Here's how the part is built. I have some questions about the finished solid (model axes, mm). Face numbers are marked on the shaded views. A direction names the side the tool comes from. Coordinates: 2 decimals unless noted, no trailing zeros. Write each loop counter-clockwise with the first axis right and the second up, starting at its lowest first coordinate (ties: lowest second). Pieces come first, ordered by that corner, then holes.
Item 1: I want a section at C-C (y = -480.5). Please give me the cut outline in (x, z), and give its area (3 significant figures).
Item 2: For the marked faces 1 and 2, which set-ups out of +Z, -Z, +X, -X, +Y, -Y let a thin tool reach every point of the face, with its end or its side?
Item 3: I want a section at D-D (z = 128.5). Please give me the cut outline in (x, y).
Item 4: Please list where these lines run through material, in increasing order: line 1 (Z direction, x = 0, y = -758); line 2 (Y direction, x = 2, z = -102.5); line 3 (Z direction, x = 10.5, y = -552).
Item 5: I'm going to push flat-ended pins straight in: P1, Ø10, axis at x = -19.5, z = -113, coming from the +Y side; P2, Ø8, axis at x = -14, y = -556.5, coming from the +Z side; P3, Ø6, axis at y = -424, z = -17.5, coming from the -X side. Where does each tip first touch, or does it pass through?
Item 6: I want a section at A-A (x = 0). Please give me the cut outline in (y, z), and give its area (3 significant figures).
Item 7: I want a section at B-B (z = 0). Please give me the cut outline in (x, y), and give its area (3 significant figures).
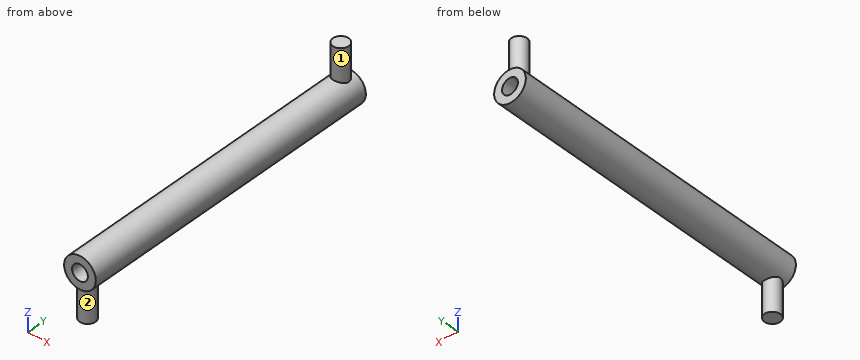
from build123d import *

# Parameters (mm, degrees)
F0_R     = 50
F0_R_2   = 25
F3_DEPTH = 1000
F4_R     = 25
F5_DEPTH = 125
F6_R     = 25
F7_DEPTH = 125


with BuildPart() as f3:
    # F0 (on Front) → F3 (new body)
    with BuildSketch(Plane.XZ):
        Circle(F0_R)
        Circle(F0_R_2, mode=Mode.SUBTRACT)
    extrude(amount=F3_DEPTH)

    # F4 (on offset) → F5 (join)
    with BuildSketch(Plane.XY.offset(-25)):
        with Locations((0, -971.540222)):
            Circle(F4_R)
    extrude(amount=-F5_DEPTH)

    # F6 (on offset) → F7 (join)
    with BuildSketch(Plane.XY.offset(25)):
        with Locations((0, -34.047124)):
            Circle(F6_R)
    extrude(amount=F7_DEPTH)


solid = f3.part
Answer:
1. outline: circle Ø100 at (0, 0); hole circle Ø50 at (0, 0)
1. area: 5,890 mm2
2. face 1: +Z
2. face 2: -Z
3. outline: circle Ø50 at (0, -34.05)
4. line 1: z = -50 to -25, 25 to 50
4. line 2: y = -996.46 to -946.62
4. line 3: z = -48.89 to -22.69, 22.69 to 48.89
5. P1: stops at y = -951.17
5. P2: stops at z = 48.99
5. P3: stops at x = -47.85
6. outline: (-1000, -50) - (-996.54, -50) - (-996.54, -150) - (-946.54, -150) - (-946.54, -50) - (0, -50) - (0, -25) - (-1000, -25) - close; (-1000, 25) - (0, 25) - (0, 50) - (-9.05, 50) - (-9.05, 150) - (-59.05, 150) - (-59.05, 50) - (-1000, 50) - close
6. area: 60,000 mm2
7. outline: (-50, -1000) - (-25, -1000) - (-25, 0) - (-50, 0) - close; (25, -1000) - (50, -1000) - (50, 0) - (25, 0) - close
7. area: 50,000 mm2
